```python
from build123d import *
from build123d.topology import SkipClean

# Parameters (mm, degrees)
SKETCH1_W               = 44.05184454
SKETCH1_H               = 18
BOSS_EXTRUDE1_DEPTH     = 1.5
SKETCH2_W               = 3
SKETCH2_H               = 18
BOSS_EXTRUDE2_DEPTH     = 13
SKETCH3_W               = 29
SKETCH3_H               = 3
BOSS_EXTRUDE3_DEPTH     = 14
CHAMFER1_SIZE           = 3
SKETCH4_R               = 3.25
CUT_EXTRUDE1_DEPTH      = 14
BOSS_EXTRUDE4_START     = 20
SKETCH5_R               = 3.25
BOSS_EXTRUDE4_DEPTH     = 20
BOSS_EXTRUDE5_START     = 7
SKETCH6_R               = 3.25
SKETCH6_W               = 22.5
SKETCH6_H               = 29
BOSS_EXTRUDE5_DEPTH     = 7
SKETCH8_R               = 3.25
BOSS_EXTRUDE6_DEPTH     = 23
BOSS_EXTRUDE8_DEPTH     = 29
SKETCH9_R               = 38.719812757
CUT_EXTRUDE2_DEPTH      = 11.5
CUT_EXTRUDE3_DEPTH      = 79.971513852
CUT_EXTRUDE3_DEPTH_BACK = 79.971513852
SKETCH10_R              = 2.5
CUT_EXTRUDE4_DEPTH      = 3
SKETCH12_R              = 3
SKETCH12_R_2            = 2.5
BOSS_EXTRUDE7_DEPTH     = 0.5
CHAMFER2_SIZE           = 0.5
SKETCH17_R              = 5.5
CUT_EXTRUDE5_DEPTH      = 6
CHAMFER3_SIZE           = 5
BOSS_EXTRUDE9_DEPTH     = 29
CHAMFER4_SIZE           = 5
SKETCH20_R              = 3.25
BOSS_EXTRUDE10_DEPTH    = 2


with BuildPart() as part:
    # Sketch1 → Boss-Extrude1 (new body)
    with BuildSketch(Plane(origin=(0, 0, 0), x_dir=(1, 0, 0), z_dir=(0, 1, 0))):
        with Locations((88.52592227, 8)):
            Rectangle(SKETCH1_W, SKETCH1_H)
        with BuildLine():
            Line((99.736944586, 5.75), (95.736944586, 5.75))
            ThreePointArc((95.736944586, 5.75), (93.486944586, 8), (95.736944586, 10.25))
            Line((95.736944586, 10.25), (99.736944586, 10.25))
            ThreePointArc((99.736944586, 10.25), (101.986944586, 8), (99.736944586, 5.75))
        make_face(mode=Mode.SUBTRACT)
    extrude(amount=BOSS_EXTRUDE1_DEPTH)

    # Sketch2 → Boss-Extrude2 (add)
    with BuildSketch(Plane(origin=(0, 1.5, 0), x_dir=(1, 0, 0), z_dir=(0, 1, 0))):
        with Locations((68, 8)):
            Rectangle(SKETCH2_W, SKETCH2_H)
    extrude(amount=BOSS_EXTRUDE2_DEPTH)

    # Sketch3 → Boss-Extrude3 (add)
    with BuildSketch(Plane.ZY.offset(-66.5)):
        with Locations((-8, 13)):
            Rectangle(SKETCH3_W, SKETCH3_H)
    extrude(amount=BOSS_EXTRUDE3_DEPTH)

    # Chamfer1
    chamfer1_edges = [part.edges().sort_by_distance(p)[0] for p in [
        (66.5, 13, 1),
        (66.5, 13, -17),
    ]]
    chamfer(chamfer1_edges, length=CHAMFER1_SIZE - 0.0001)  # a hair under: the kernel refuses the full size

    # Sketch4 → Cut-Extrude1 (cut)
    with BuildSketch(Plane(origin=(0, 14.5, 0), x_dir=(1, 0, 0), z_dir=(0, 1, 0))):
        with Locations(Location((60, 16, 0), (0, 0, 270))):
            Circle(SKETCH4_R)
        with Locations(Location((60, 0, 0), (0, 0, 270))):
            Circle(SKETCH4_R)
    extrude(amount=-CUT_EXTRUDE1_DEPTH, mode=Mode.SUBTRACT)

    # Sketch5 → Boss-Extrude4 (add)
    with SkipClean():  # the faces are left unmerged after this step: merging them gives an invalid solid
        with BuildSketch(Plane(origin=(0, 14.5, 0), x_dir=(1, 0, 0), z_dir=(0, 1, 0)).offset(BOSS_EXTRUDE4_START)):
            Polygon((69.5, -1), (69.5, 17), (66.5, 20), (66.5, 22.5), (52.5, 22.5), (52.5, -6.5), (66.5, -6.5), (66.5, -4), align=None)
            with Locations(Location((60, 16, 0), (0, 0, 270))):
                Circle(SKETCH5_R, mode=Mode.SUBTRACT)
            with Locations(Location((60, 0, 0), (0, 0, 270))):
                Circle(SKETCH5_R, mode=Mode.SUBTRACT)
        extrude(amount=-BOSS_EXTRUDE4_DEPTH)

    # Sketch6 → Boss-Extrude5 (add)
    # profile 1 of 3: a face of its own
    with BuildSketch(Plane(origin=(0, 34.5, 0), x_dir=(1, 0, 0), z_dir=(0, 1, 0)).offset(BOSS_EXTRUDE5_START)):
        Polygon((30, -6.5), (30, 22.5), (7.5, 22.5), (-6.5, 22.5), (-6.5, 20), (-9.5, 17), (-9.5, -1), (-6.5, -4), (-6.5, -6.5), (7.5, -6.5), align=None)
        with Locations(Location((0, 0, 0), (0, 0, 90))):
            Circle(SKETCH6_R, mode=Mode.SUBTRACT)
        with Locations(Location((0, 16, 0), (0, 0, 90))):
            Circle(SKETCH6_R, mode=Mode.SUBTRACT)
    # profile 2 of 3: a face of its own
    with BuildSketch(Plane(origin=(0, 34.5, 0), x_dir=(1, 0, 0), z_dir=(0, 1, 0)).offset(BOSS_EXTRUDE5_START)):
        with Locations((41.25, 8)):
            Rectangle(SKETCH6_W, SKETCH6_H)
    # profile 3 of 3: a face of its own
    with BuildSketch(Plane(origin=(0, 34.5, 0), x_dir=(1, 0, 0), z_dir=(0, 1, 0)).offset(BOSS_EXTRUDE5_START)):
        Polygon((66.5, -6.5), (66.5, -4), (69.5, -1), (69.5, 17), (66.5, 20), (66.5, 22.5), (52.5, 22.5), (52.5, -6.5), align=None)
        with Locations(Location((60, 0, 0), (0, 0, 270))):
            Circle(SKETCH6_R, mode=Mode.SUBTRACT)
        with Locations(Location((60, 16, 0), (0, 0, 270))):
            Circle(SKETCH6_R, mode=Mode.SUBTRACT)
    extrude(amount=-BOSS_EXTRUDE5_DEPTH)

    # Sketch8 → Boss-Extrude6 (add)
    with BuildSketch(Plane.XZ.offset(-34.5)):
        Polygon((7.5, -22.5), (7.5, 6.5), (-6.5, 6.5), (-6.5, 4), (-9.5, 1), (-9.5, -17), (-6.5, -20), (-6.5, -22.5), align=None)
        with Locations(Location((0, -16, 0), (0, 0, 270))):
            Circle(SKETCH8_R, mode=Mode.SUBTRACT)
        with Locations(Location((0, 0, 0), (0, 0, 270))):
            Circle(SKETCH8_R, mode=Mode.SUBTRACT)
    extrude(amount=BOSS_EXTRUDE6_DEPTH)

    # Sketch18 → Boss-Extrude8 (add)
    with BuildSketch(Plane.XY.offset(6.5)):
        Polygon((9.5, 60.5), (29.5, 60.5), (29.5, 41.5), (34.5, 41.5), (34.5, 63.5), (9.5, 63.5), align=None)
    extrude(amount=-BOSS_EXTRUDE8_DEPTH)

    # Sketch9 → Cut-Extrude2 (cut)
    with BuildSketch(Plane(origin=(0, 0, 0), x_dir=(-1, 0, 0), z_dir=(0, -1, 0))):
        with Locations((-87.720791246, 8.661967718)):
            Circle(SKETCH9_R)
    extrude(amount=-CUT_EXTRUDE2_DEPTH, mode=Mode.SUBTRACT)

    # Sketch10 → Cut-Extrude3 (cut, two sides: drawn at the far end of the back side and taken through both)
    with BuildSketch(Plane(origin=(0, 41.5, 0), x_dir=(1, 0, 0), z_dir=(0, 1, 0)).offset(-CUT_EXTRUDE3_DEPTH_BACK)):
        with Locations(Location((18, 8, 0), (0, 0, 270))):
            Circle(SKETCH10_R)
    extrude(amount=CUT_EXTRUDE3_DEPTH + CUT_EXTRUDE3_DEPTH_BACK, mode=Mode.SUBTRACT)

    # Sketch11 → Cut-Extrude4 (cut)
    with BuildSketch(Plane(origin=(0, 34.5, 0), x_dir=(-1, 0, 0), z_dir=(0, -1, 0))):
        Polygon((-18, 3.381197846), (-14, 5.690598923), (-14, 10.309401077), (-18, 12.618802154), (-22, 10.309401077), (-22, 5.690598923), align=None)
    extrude(amount=-CUT_EXTRUDE4_DEPTH, mode=Mode.SUBTRACT)

    # Sketch12 → Boss-Extrude7 (add)
    with BuildSketch(Plane(origin=(0, 41.5, 0), x_dir=(1, 0, 0), z_dir=(0, 1, 0))):
        with Locations(Location((18, 8, 0), (0, 0, 270))):
            Circle(SKETCH12_R)
        with Locations(Location((18, 8, 0), (0, 0, 270))):
            Circle(SKETCH12_R_2, mode=Mode.SUBTRACT)
    extrude(amount=BOSS_EXTRUDE7_DEPTH)

    # Chamfer2
    chamfer2_edges = [part.edges().sort_by_distance(p)[0] for p in [
        (18, 41.5, -11),
    ]]
    chamfer(chamfer2_edges, length=CHAMFER2_SIZE - 0.0001)  # a hair under: the kernel refuses the full size

    # Sketch17 → Cut-Extrude5 (cut)
    with BuildSketch(Plane(origin=(0, 41.5, 0), x_dir=(1, 0, 0), z_dir=(0, 1, 0))):
        with Locations(Location((0, 16, 0), (0, 0, 270))):
            Circle(SKETCH17_R)
        with Locations(Location((0, 0, 0), (0, 0, 270))):
            Circle(SKETCH17_R)
    extrude(amount=-CUT_EXTRUDE5_DEPTH, mode=Mode.SUBTRACT)

    # Chamfer3
    chamfer3_edges = [part.edges().sort_by_distance(p)[0] for p in [
        (9.5, 62, -22.5),
        (9.5, 62, 6.5),
    ]]
    chamfer(chamfer3_edges, length=CHAMFER3_SIZE)

    # Sketch19 → Boss-Extrude9 (add)
    with BuildSketch(Plane.XY.offset(6.5)):
        Polygon((34.5, 63.5), (52.5, 63.5), (52.5, 41.5), (49.5, 41.5), (49.5, 60.5), (29.5, 60.5), align=None)
    extrude(amount=-BOSS_EXTRUDE9_DEPTH)

    # Chamfer4
    chamfer4_edges = [part.edges().sort_by_distance(p)[0] for p in [
        (52.5, 63.5, -8),
        (49.5, 60.5, -8),
    ]]
    chamfer(chamfer4_edges, length=CHAMFER4_SIZE)

    # Sketch20 → Boss-Extrude10 (add)
    # profile 1 of 2: a face of its own
    with SkipClean():  # the faces are left unmerged after this step: merging them gives an invalid solid
        with BuildSketch(Plane.XZ.offset(-11.5)):
            Polygon((66.5, -20), (69.5, -17), (69.5, 1), (66.5, 4), (66.5, 6.5), (52.5, 6.5), (52.5, -22.5), (66.5, -22.5), align=None)
            with Locations(Location((60, 0, 0), (0, 0, 90))):
                Circle(SKETCH20_R, mode=Mode.SUBTRACT)
            with Locations(Location((60, -16, 0), (0, 0, 90))):
                Circle(SKETCH20_R, mode=Mode.SUBTRACT)
        # profile 2 of 2: a face of its own
        with BuildSketch(Plane.XZ.offset(-11.5)):
            Polygon((7.5, -22.5), (7.5, 6.5), (-6.5, 6.5), (-6.5, 4), (-9.5, 1), (-9.5, -17), (-6.5, -20), (-6.5, -22.5), align=None)
            with Locations(Location((0, 0, 0), (0, 0, 270))):
                Circle(SKETCH20_R, mode=Mode.SUBTRACT)
            with Locations(Location((0, -16, 0), (0, 0, 270))):
                Circle(SKETCH20_R, mode=Mode.SUBTRACT)
        extrude(amount=BOSS_EXTRUDE10_DEPTH)


solid = part.part
```
Geometry check sheet. Reference: the model listing, model coordinates, mm. A direction names the side the tool comes from. Round coordinates to 2 decimals unless told otherwise and drop trailing zeros. Loops run counter-clockwise (first coordinate to the right, second up) from the corner with the lowest first, then second, coordinate; pieces in that order, holes last. Notation, with made-up numbers: (88.25, 46.5) - (121.25, 46.5) arc R17 cw to (121.25, 58.5) - close; hole circle Ø6 at (59, 14.5). An arc over 180 degrees is marked (long way). Write item = value, one per line. Start each with the question number.
1. Section check C-C on x = 46.5. Enter the section's corners in (y, z).
2. Mould release check, pull along Z, two halves, no side actions. Record for faces 1 (the face through (56.778, 25.724, -16.423)), 2 (the face through (34.5, 51, -8)), 3 (the face through (12, 62, -20)), 4 (the face through (-4, 35.5, -16)): released by +Z, released by -Z, zero draft, split by the parting line, or undercut.
3. Thickness scan on line 1 (Z direction, x = 0, y = 17.75); line 2 (X direction, y = 37.95, z = 0); line 3 (X direction, y = 28, z = 0). Record the ranges inside material, lowest first.
4. Section check B-B on y = 33.5. Enter the section's corners in (x, z).
5. Section check A-A on z = 0. Give the number of separate pieces and of enclosed holes in the cut face, then the cut area to 3 significant figures.
6. Section check D-D on x = 0. Enter the section's corners in (y, z), then the cut area to 3 significant figures.
7. Set-up check for faces 5 (the face through (7.5, 22, -8)), 6 (the face through (61, 41.5, -8)), 7 (the face through (49.5, 48, -8)): record each of +Z, -Z, +X, -X, +Y, -Y from which the full face is reachable in a straight line by a thin tool's end or side.
8. Depth check by flat-ended pin: pin 1 (2.5 mm diameter, centred on x = 16, z = -9, fed in from -Y); pin 2 (14.5 mm diameter, centred on x = 0, z = -16, fed in from -Y); pin 3 (6 mm diameter, centred on y = 51, z = -1, fed in from +X); pin 4 (9 mm diameter, centred on x = 0, z = 0, fed in from +Y). Enter the tip coordinate at first touch or a pass-through.
Working result:
q1.outline = (34.5, -22.5) - (41.5, -22.5) - (41.5, 6.5) - (34.5, 6.5) - close; (58.5, -22.5) - (63.5, -22.5) - (63.5, 6.5) - (58.5, 6.5) - close
q2.face_1 = undercut
q2.face_2 = zero draft
q2.face_3 = released by -Z
q2.face_4 = undercut
q3.line_1 = -22.5 to -19.25, -12.75 to -3.25, 3.25 to 6.5
q3.line_2 = -9.5 to -5.5, 5.5 to 56.75, 63.25 to 69.5
q3.line_3 = -9.5 to -3.25, 3.25 to 7.5, 52.5 to 56.75, 63.25 to 69.5
q4.outline = (-9.5, -17) - (-6.5, -20) - (-6.5, -22.5) - (7.5, -22.5) - (7.5, 6.5) - (-6.5, 6.5) - (-6.5, 4) - (-9.5, 1) - close; (52.5, -22.5) - (66.5, -22.5) - (66.5, -20) - (69.5, -17) - (69.5, 1) - (66.5, 4) - (66.5, 6.5) - (52.5, 6.5) - close; hole circle Ø6.5 at (0, -16); hole circle Ø6.5 at (0, 0); hole circle Ø6.5 at (60, -16); hole circle Ø6.5 at (60, 0)
q5.separate_pieces = 3
q5.enclosed_holes = 1
q5.area = 1,240 mm^2
q6.outline = (9.5, -22.5) - (41.5, -22.5) - (41.5, -21.5) - (35.5, -21.5) - (35.5, -19.25) - (9.5, -19.25) - close; (9.5, -12.75) - (35.5, -12.75) - (35.5, -10.5) - (41.5, -10.5) - (41.5, -5.5) - (35.5, -5.5) - (35.5, -3.25) - (9.5, -3.25) - close; (9.5, 3.25) - (35.5, 3.25) - (35.5, 5.5) - (41.5, 5.5) - (41.5, 6.5) - (9.5, 6.5) - close
q6.area = 458 mm^2
q7.face_5 = +Z, -Z, -Y
q7.face_6 = +Z, -Z, +X, +Y
q7.face_7 = +Z, -Z
q8.pin_1 = 37.5
q8.pin_2 = 9.5
q8.pin_3 = 52.5
q8.pin_4 = 35.5
